from build123d import *

# Parameters (mm, degrees)
F1_DEPTH = 100


with BuildPart() as f1:
    # F0 (on Front) → F1 (new body)
    with BuildSketch(Plane.XZ):
        Polygon((65.12177, 17.418353), (45.366846, 49.860738), (11.208269, 66.472691), (-26.508854, 61.980034), (-55.809603, 37.809154), (-67.391198, 1.634135), (-57.576563, -35.05971), (-29.481777, -60.622346), (7.973266, -66.937814), (42.896852, -52.001), (64.200992, -20.554235), align=None)
    extrude(amount=-F1_DEPTH)


solid = f1.part
Design review of the part built by this model. Coordinates are the model's own, in mm. Round coordinates to 2 decimals unless told otherwise and drop trailing zeros. Write each loop counter-clockwise with the first axis right and the second up, starting at its lowest first coordinate (ties: lowest second). Pieces come first, ordered by that corner, then holes.
Item 1: Draft analysis for pull direction X (two halves, no side actions). For faces 1 (the flat face through (-40.954, 49.3, 50.064)), 2 (the flat face through (-2, 0, 1)), 3 (the flat face through (55.383, 49.3, 33.412)), state which applies: released by +X, released by -X, zero draft, split by the parting line, or undercut.
Item 2: Consider section A-A on y = 86. Give the boundary of the cut face in (x, z), and give its area (3 significant figures).
Item 3: Consider section B-B on x = 40. Give the boundary of the cut face in (y, z).
Item 4: For pin 1 Ø8 at (y, z) = (79.5, 19.5) entering from -X; pin 2 Ø1 at (x, y) = (51.5, 87) entering from +Z; pin 3 Ø8 at (y, z) = (39, 50) entering from +X, all flat-tipped, find the tip position at first contact; note any pin that passes through.
Item 5: Consider section C-C on z = 54. Give the boundary of the cut face in (x, y), and give its area (3 significant figures).
Item 6: Wall thickness on L1, parallel to X at y = 27.5, z = 49; L2, parallel to Z at x = 9, y = 57.5; L3, parallel to Z at x = -14.5, y = 9.5: over which ranges is each line inside the solid? List them lowest first.
Check values:
1. face 1: released by -X
1. face 2: zero draft
1. face 3: released by +X
2. outline: (-67.39, 1.63) - (-57.58, -35.06) - (-29.48, -60.62) - (7.97, -66.94) - (42.9, -52) - (64.2, -20.55) - (65.12, 17.42) - (45.37, 49.86) - (11.21, 66.47) - (-26.51, 61.98) - (-55.81, 37.81) - close
2. area: 13,500 mm2
3. outline: (0, -53.24) - (100, -53.24) - (100, 52.47) - (0, 52.47) - close
4. pin 1: stops at x = -62.95
4. pin 2: stops at z = 40.61
4. pin 3: stops at x = 47.72
5. outline: (-36.18, 0) - (36.86, 0) - (36.86, 100) - (-36.18, 100) - close
5. area: 7,300 mm2
6. L1: x = -42.24 to 45.89
6. L2: z = -66.5 to 66.21
6. L3: z = -63.15 to 63.41
